For this review, take the finished solid that the model builds, in its own axes (mm). Face numbers are marked on the shaded views. A direction names the side the tool comes from. Round coordinates to 2 decimals unless told otherwise and drop trailing zeros. Loops run counter-clockwise (first coordinate to the right, second up) from the corner with the lowest first, then second, coordinate; pieces in that order, holes last. Notation, with made-up numbers: M 63.25,35 L 102.25,35 A10 ccw 102.25,48 Z; hole C 5,28 d4. An arc over 180 degrees is marked long. Write item = value, one per line. Start each with the question number.
```python
from build123d import *

# Parameters (mm, degrees)
SKETCH_1_R          = 4.5
EXTRUDE_2_DEPTH     = 5
FILLET1_R           = 20
SKETCH_1_5_W        = 12
SKETCH_1_5_H        = 11.85
SKETCH_1_5_R        = 4.5
SKETCH_1_5_R_2      = 2.5
BOSS_EXTRUDE1_DEPTH = 3.85
BOSS_EXTRUDE3_DEPTH = 5
SKETCH1_3_W         = 100
SKETCH1_3_H         = 10
BOSS_EXTRUDE4_DEPTH = 30
SKETCH2_W           = 100
SKETCH2_H           = 10
SKETCH2_R           = 2.4
BOSS_EXTRUDE5_DEPTH = 5
FILLET2_R           = 5


with BuildPart() as part:
    # Sketch 1 → Extrude 2 (new body)
    with BuildSketch(Plane.XY):
        with BuildLine():
            ThreePointArc((-50, -48.989794856), (0, -70), (50, -48.989794856))
            Line((50, -48.989794856), (50, 48.989794856))
            ThreePointArc((50, 48.989794856), (0, 70), (-50, 48.989794856))
            Line((-50, 48.989794856), (-50, -48.989794856))
        make_face()
        with BuildLine():
            ThreePointArc((27.5, -17.5), (24.571067812, -24.571067812), (17.5, -27.5))
            Line((17.5, -27.5), (-17.5, -27.5))
            ThreePointArc((-17.5, -27.5), (-24.571067812, -24.571067812), (-27.5, -17.5))
            Line((-27.5, -17.5), (-27.5, 17.5))
            ThreePointArc((-27.5, 17.5), (-24.571067812, 24.571067812), (-17.5, 27.5))
            Line((-17.5, 27.5), (17.5, 27.5))
            ThreePointArc((17.5, 27.5), (24.571067812, 24.571067812), (27.5, 17.5))
            Line((27.5, 17.5), (27.5, -17.5))
        make_face(mode=Mode.SUBTRACT)
        with Locations((39, -39)):
            Circle(SKETCH_1_R, mode=Mode.SUBTRACT)
        with Locations((-39, -39)):
            Circle(SKETCH_1_R, mode=Mode.SUBTRACT)
        with Locations((39, 39)):
            Circle(SKETCH_1_R, mode=Mode.SUBTRACT)
        with Locations((-39, 39)):
            Circle(SKETCH_1_R, mode=Mode.SUBTRACT)
    extrude(amount=EXTRUDE_2_DEPTH)

    # Fillet1
    fillet1_edges = [part.edges().sort_by_distance(p)[0] for p in [
        (-50, 48.989794856, 2.5),
        (50, 48.989794856, 2.5),
        (50, -48.989794856, 2.5),
        (-50, -48.989794856, 2.5),
    ]]
    fillet(fillet1_edges, radius=FILLET1_R)

    # Sketch 1_5 → Boss-Extrude1 (add)
    with BuildSketch(Plane.XY):
        with Locations((39, -39)):
            Rectangle(SKETCH_1_5_W, SKETCH_1_5_H)
        with Locations((39, -39)):
            Circle(SKETCH_1_5_R, mode=Mode.SUBTRACT)
        with Locations((-39, -39)):
            Rectangle(SKETCH_1_5_W, SKETCH_1_5_H)
        with Locations((-39, -39)):
            Circle(SKETCH_1_5_R, mode=Mode.SUBTRACT)
        with Locations((-39, 39)):
            Rectangle(SKETCH_1_5_W, SKETCH_1_5_H)
        with Locations((-39, 39)):
            Circle(SKETCH_1_5_R, mode=Mode.SUBTRACT)
        with Locations((39, 39)):
            Rectangle(SKETCH_1_5_W, SKETCH_1_5_H)
        with Locations((39, 39)):
            Circle(SKETCH_1_5_R, mode=Mode.SUBTRACT)
        with Locations((39, 39)):
            Circle(SKETCH_1_5_R)
        with Locations((39, 39)):
            Circle(SKETCH_1_5_R_2, mode=Mode.SUBTRACT)
        with Locations((-39, 39)):
            Circle(SKETCH_1_5_R)
        with Locations((-39, 39)):
            Circle(SKETCH_1_5_R_2, mode=Mode.SUBTRACT)
        with Locations((-39, -39)):
            Circle(SKETCH_1_5_R)
        with Locations((-39, -39)):
            Circle(SKETCH_1_5_R_2, mode=Mode.SUBTRACT)
        with Locations((39, -39)):
            Circle(SKETCH_1_5_R)
        with Locations((39, -39)):
            Circle(SKETCH_1_5_R_2, mode=Mode.SUBTRACT)
    extrude(amount=-BOSS_EXTRUDE1_DEPTH)

    # Sketch1 → Boss-Extrude3 (add)
    with BuildSketch(Plane.XY):
        with BuildLine():
            Line((50, -84), (50, -40))
            ThreePointArc((50, -40), (0, -60.710678119), (-50, -40))
            Line((-50, -40), (-50, -84))
            Line((-50, -84), (50, -84))
        make_face()
    extrude(amount=BOSS_EXTRUDE3_DEPTH)

    # Sketch1_3 → Boss-Extrude4 (add)
    with BuildSketch(Plane.XY):
        with Locations((0, -89)):
            Rectangle(SKETCH1_3_W, SKETCH1_3_H)
    extrude(amount=BOSS_EXTRUDE4_DEPTH)

    # Sketch2 → Boss-Extrude5 (add)
    with BuildSketch(Plane.XY.offset(30)):
        with BuildLine():
            ThreePointArc((-15, -4), (0, 4.027756377), (15, -4))
            Line((15, -4), (50, -64))
            Line((50, -64), (50, -84))
            Line((50, -84), (-50, -84))
            Line((-50, -84), (-50, -64))
            Line((-50, -64), (-15, -4))
        make_face()
        Polygon((4, -11.690598923), (0, -9.381197846), (-4, -11.690598923), (-4, -16.309401077), (0, -18.618802154), (4, -16.309401077), align=None, mode=Mode.SUBTRACT)
        Polygon((-35, -61.690598923), (-39, -59.381197846), (-43, -61.690598923), (-43, -66.309401077), (-39, -68.618802154), (-35, -66.309401077), align=None, mode=Mode.SUBTRACT)
        Polygon((35, -61.690598923), (39, -59.381197846), (43, -61.690598923), (43, -66.309401077), (39, -68.618802154), (35, -66.309401077), align=None, mode=Mode.SUBTRACT)
        with Locations((0, -89)):
            Rectangle(SKETCH2_W, SKETCH2_H)
        Polygon((39, -59.381197846), (43, -61.690598923), (43, -66.309401077), (39, -68.618802154), (35, -66.309401077), (35, -61.690598923), align=None)
        with Locations((39, -64)):
            Circle(SKETCH2_R, mode=Mode.SUBTRACT)
        Polygon((4, -16.309401077), (4, -11.690598923), (0, -9.381197846), (-4, -11.690598923), (-4, -16.309401077), (0, -18.618802154), align=None)
        with Locations((0, -14)):
            Circle(SKETCH2_R, mode=Mode.SUBTRACT)
        Polygon((-35, -66.309401077), (-35, -61.690598923), (-39, -59.381197846), (-43, -61.690598923), (-43, -66.309401077), (-39, -68.618802154), align=None)
        with Locations((-39, -64)):
            Circle(SKETCH2_R, mode=Mode.SUBTRACT)
    extrude(amount=BOSS_EXTRUDE5_DEPTH)

    # Fillet2
    fillet2_edges = [part.edges().sort_by_distance(p)[0] for p in [
        (0, -84, 5),
        (0, -84, 30),
        (0, -94, 0),
        (0, -94, 35),
    ]]
    fillet(fillet2_edges, radius=FILLET2_R)


solid = part.part
```
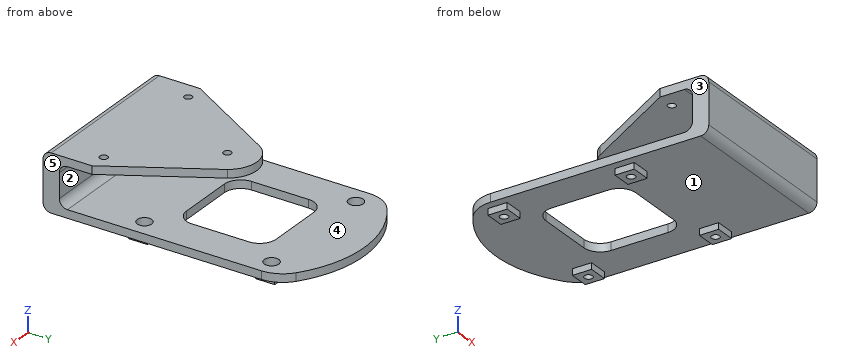
(1) Add section C-C on x = -11. Write out the cut boundary in (y, z), and give its area (3 significant figures).
(2) Add section B-B on z = 3. Write out the cut boundary in (x, y), and give its area (3 significant figures).
(3) Draft analysis for pull direction X (two halves, no side actions). For the marked faces 1, 2 and 3, state which applies: +X half, -X half, draft (parallel to the pull), parting line (faces both ways), or undercut.
(4) Add section A-A on x = 0. Write out the cut boundary in (y, z).
(5) For pin 1 Ø10.5 at (x, y) = (-39, 39) entering from -Z; pin 2 Ø1.2 at (x, z) = (-40.5, -2) entering from +Y (3 decimals); pin 3 Ø5 at (x, z) = (-19.5, 26) entering from +Y; pin 4 Ø10 at (x, z) = (38.5, 15.5) entering from +Y, all flat-tipped, find the tip position at first contact; note any pin that passes through.
(6) Wall thickness on L1, parallel to Y at x = 39, z = 3; L2, parallel to Z at x = 6.5, y = -50; L3, parallel to Y at x = 40, z = 4: over which ranges is each line inside the solid? List them lowest first.
(7) Tool access review of the marked faces 4 and 5: name each direction out of +Z, -Z, +X, -X, +Y, -Y from which nothing blocks a thin tool from reaching the whole face with its end or side.
(8) Add section D-D on y = -14. Write out the cut boundary in (x, z).
Answer sheet:
q1.outline = M -94,5 A5 ccw -89,0 L -27.5,0 L -27.5,5 L -79,5 A5 cw -84,10 L -84,25 A5 cw -79,30 L 0.28,30 L 0.28,35 L -89,35 A5 ccw -94,30 Z; M 27.5,0 L 69.13,0 L 69.13,5 L 27.5,5 Z
q1.area = 1,260 mm²
q2.outline = M -50,-93.58 L 50,-93.58 L 50,40 A20 ccw 42,56 A70 ccw -42,56 A20 ccw -50,40 Z; hole C -39,-39 d9; hole C -39,39 d9; hole M -27.5,-17.5 A10 ccw -17.5,-27.5 L 17.5,-27.5 A10 ccw 27.5,-17.5 L 27.5,17.5 A10 ccw 17.5,27.5 L -17.5,27.5 A10 ccw -27.5,17.5 Z; hole C 39,-39 d9; hole C 39,39 d9
q2.area = 12,500 mm²
q3.face_1 = undercut
q3.face_2 = draft
q3.face_3 = -X half
q4.outline = M -94,5 A5 ccw -89,0 L -27.5,0 L -27.5,5 L -79,5 A5 cw -84,10 L -84,25 A5 cw -79,30 L -16.4,30 L -16.4,35 L -89,35 A5 ccw -94,30 Z; M -11.6,30 L 4.03,30 L 4.03,35 L -11.6,35 Z; M 27.5,0 L 70,0 L 70,5 L 27.5,5 Z
q5.pin_1 = -3.85
q5.pin_2 = 44.925
q5.pin_3 = -82.57
q5.pin_4 = -84
q6.L1 = -93.58 to -43.5, -34.5 to 34.5, 43.5 to 58.13
q6.L2 = 0 to 5, 30 to 35
q6.L3 = -93.9 to -43.39, -34.61 to 34.61, 43.39 to 57.45
q7.face_4 = +X, -X, +Y
q7.face_5 = +Z, -Z, +X, +Y, -Y
q8.outline = M -50,0 L -27.5,0 L -27.5,5 L -50,5 Z; M -20.83,30 L -2.4,30 L -2.4,35 L -20.83,35 Z; M 2.4,30 L 20.83,30 L 20.83,35 L 2.4,35 Z; M 27.5,0 L 50,0 L 50,5 L 27.5,5 Z
